```python
from build123d import *

# Parameters (mm, degrees)
SKETCH2_W             = 15
SKETCH2_H             = 20
BOSS_EXTRUDE1_DEPTH   = 15
BOSS_EXTRUDE1_2_DEPTH = 15
BOSS_EXTRUDE2_DEPTH   = 35
SKETCH9_R             = 6
BOSS_EXTRUDE6_DEPTH   = 15
HOLE1_D               = 15
HOLE1_DEPTH           = 99.968745116
HOLE1_CBORE_D         = 20
HOLE1_CBORE_DEPTH     = 5


with BuildPart() as part:
    # Sketch2 → Boss-Extrude1 (new body)
    with BuildSketch(Plane.XY):
        with Locations((7.5, 10)):
            Rectangle(SKETCH2_W, SKETCH2_H)
    extrude(amount=BOSS_EXTRUDE1_DEPTH)



with BuildPart() as body_2:
    # Sketch2 → Boss-Extrude1 2 (new body)
    with BuildSketch(Plane.XY):
        Polygon((45, 20), (45, 0), (55, 0), (55, 5), (100, 5), (100, 20), align=None)
    extrude(amount=BOSS_EXTRUDE1_2_DEPTH)


with BuildPart() as part_1:
    add(part.part)

    add(body_2.part)  # Boss-Extrude2 merges body 2
    # Sketch3 → Boss-Extrude2 (add)
    with BuildSketch(Plane.XY):
        Polygon((100, 20), (100, 5), (55, 5), (55, 0), (0, 0), (0, 20), align=None)
    extrude(amount=-BOSS_EXTRUDE2_DEPTH)

    # Sketch9 → Boss-Extrude6 (add)
    with BuildSketch(Plane.XY):
        with BuildLine():
            Line((40, 45), (10, 45))
            ThreePointArc((10, 45), (2.928932188, 42.071067812), (0, 35))
            Line((0, 35), (0, 20))
            Line((0, 20), (57.320508076, 20))
            ThreePointArc((57.320508076, 20), (54.820508076, 20.669872981), (52.990381057, 22.5))
            Line((52.990381057, 22.5), (40, 45))
        make_face()
        with Locations((15, 33)):
            Circle(SKETCH9_R, mode=Mode.SUBTRACT)
    extrude(amount=-BOSS_EXTRUDE6_DEPTH)

    # Hole1
    with Locations(Plane(origin=(0, 20, 0), x_dir=(1, 0, 0), z_dir=(0, 1, 0))):
        with Locations((80, 10)):
            CounterBoreHole(HOLE1_D / 2, HOLE1_CBORE_D / 2, HOLE1_CBORE_DEPTH, depth=HOLE1_DEPTH)


solid = part_1.part
```
Here's how the part is built. I have some questions about the finished solid (model axes, mm). A direction names the side the tool comes from. Coordinates: 2 decimals unless noted, no trailing zeros. Loops run counter-clockwise (first coordinate to the right, second up) from the corner with the lowest first, then second, coordinate; pieces in that order, holes last. Notation, with made-up numbers: (25, 76) - (39, 76) arc R8 ccw to (39, 82) - close; hole circle Ø2 at (-4, 27). An arc over 180 degrees is marked (long way). Return JSON: item names as keys, results as strings. Group by question number.
Item 1: I need wall thicknesses on line 1 (Y direction, x = 17.5, z = -19.5); line 2 (Z direction, x = 20, y = 24); line 3 (Z direction, x = 80, y = 17.75). Which ranges of each line are inside material? Lowest first, please. Write a range as from..to.
Item 2: If we section it at B-B on y = 12: Write out the boundary of the cut face in (x, z), and give its area (3 significant figures).
Item 3: On a 3-axis mill with a long thin cutter (end or side, diameter ignored), from which of +Z, -Z, +X, -X, +Y, -Y can I reach the whole of each face in a straight line? I mean faces 1 (the face through (22, 33, -15)), 2 (the face through (55, 3, -10)), 3 (the face through (84, 15, -17)). Say none if no direction works.
Item 4: We'd pull the mould along Z, two halves only. Please class faces 4 (the face through (7, 20, 8)), 5 (the face through (70, 18, -10)), 6 (the face through (7, 10, 15)): +Z half, -Z half, draft (parallel to the pull), parting line (faces both ways), or undercut.
Item 5: If we section it at A-A on z = 5: Write out the boundary of the cut face in (x, y).
Item 6: Will these pins go through, and if not, where does the flat tip stop? P1, Ø7, axis at x = 15, y = 33, coming from the +Z side; P2, Ø23, axis at x = 80, z = -10, coming from the -Y side; P3, Ø6, axis at x = 84.5, z = -19, coming from the +Y side; P4, Ø7.5, axis at x = 29, y = 26.5, coming from the -Z side.
Item 7: If we section it at D-D on x = 80: Write out the boundary of the cut face in (y, z), and give its area (3 significant figures).
Item 8: If we section it at C-C on z = -6: Write out the boundary of the cut face in (x, y).
Calculated:
{
 "1": {"line 1": "y = 0..20", "line 2": "z = -15..0", "line 3": "z = -35..-20, 0..15"},
 "2": {"outline": "(0, -35) - (100, -35) - (100, 15) - (45, 15) - (45, 0) - (15, 0) - (15, 15) - (0, 15) - close; hole circle Ø15 at (80, -10)", "area": "4,370 mm^2"},
 "3": {"face 1": "-Z, +X, -X, +Y", "face 2": "+Z, -Z, +X, -Y", "face 3": "+Y"},
 "4": {"face 4": "draft", "face 5": "undercut", "face 6": "+Z half"},
 "5": {"outline": "(0, 0) - (15, 0) - (15, 20) - (0, 20) - close; (45, 0) - (55, 0) - (55, 5) - (100, 5) - (100, 20) - (45, 20) - close"},
 "6": {"P1": "passes through", "P2": "stops at y = 5", "P3": "stops at y = 20", "P4": "stops at z = -15"},
 "7": {"outline": "(5, -35) - (20, -35) - (20, -20) - (15, -20) - (15, -17.5) - (5, -17.5) - close; (5, -2.5) - (15, -2.5) - (15, 0) - (20, 0) - (20, 15) - (5, 15) - close", "area": "500 mm^2"},
 "8": {"outline": "(0, 0) - (55, 0) - (55, 5) - (73.66, 5) - (73.66, 15) - (70.83, 15) - (70.83, 20) - (57.32, 20) arc R5 cw to (52.99, 22.5) - (40, 45) - (10, 45) arc R10 ccw to (0, 35) - close; (86.34, 5) - (100, 5) - (100, 20) - (89.17, 20) - (89.17, 15) - (86.34, 15) - close; hole circle Ø12 at (15, 33)"}
}
